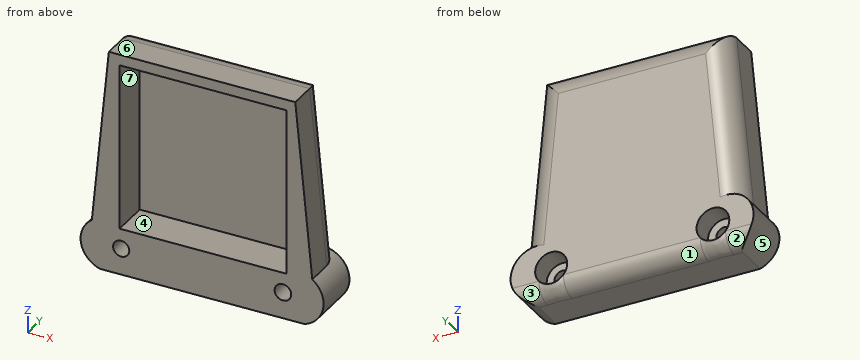
from build123d import *

# Parameters (mm, degrees)
SKETCH_R        = 1.501869
SKETCH_R_2      = 1.541907
PAD_DEPTH       = 9
SKETCH003_W     = 31
SKETCH003_H     = 31
POCKET_DEPTH    = 7
FILLET_R        = 4
SKETCH004_R     = 2.968472
SKETCH004_R_2   = 3.036595
POCKET001_DEPTH = 4
FILLET001_R     = 3


with BuildPart() as part:
    # Sketch → Pad (new body)
    with BuildSketch(Plane.XZ):
        with BuildLine():
            ThreePointArc((2.716597, 148.883863), (0.695773, 143.988618), (4.206694, 140.023699))
            Line((4.206694, 140.023699), (42.11266, 140.023699))
            ThreePointArc((42.11266, 140.023699), (45.623581, 143.988618), (43.602757, 148.883863))
            Line((40.447369, 181.653), (43.602757, 148.883863))
            Line((5.871985, 181.653), (40.447369, 181.653))
            Line((2.716597, 148.883863), (5.871985, 181.653))
        make_face()
        with Locations((8.159677, 144.938485)):
            Circle(SKETCH_R, mode=Mode.SUBTRACT)
        with Locations((38.159677, 144.938485)):
            Circle(SKETCH_R_2, mode=Mode.SUBTRACT)
    extrude(amount=PAD_DEPTH)

    # Sketch003 (on Face10 of Pad) → Pocket (cut)
    with BuildSketch(Plane.XZ.offset(9)):
        with Locations((23.362282, 164.148895)):
            Rectangle(SKETCH003_W, SKETCH003_H)
    extrude(amount=-POCKET_DEPTH, mode=Mode.SUBTRACT)

    # Fillet
    fillet_edges = [part.edges().sort_by_distance(p)[0] for p in [
        (42.025063, 0, 165.268432),
        (23.159677, 0, 181.653),
        (4.294291, 0, 165.268432),
    ]]
    fillet(fillet_edges, radius=FILLET_R)

    # Sketch004 (on Face5 of Fillet) → Pocket001 (cut)
    with BuildSketch(Plane(origin=(0, 0, 0), x_dir=(1, 0, 0), z_dir=(0, 1, 0))):
        with Locations((38.159676, -144.938507)):
            Circle(SKETCH004_R)
        with Locations((8.159677, -144.938507)):
            Circle(SKETCH004_R_2)
    extrude(amount=-POCKET001_DEPTH, mode=Mode.SUBTRACT)

    # Fillet001
    fillet001_edges = [part.edges().sort_by_distance(p)[0] for p in [
        (23.159677, 0, 140.023699),
    ]]
    fillet(fillet001_edges, radius=FILLET001_R)


solid = part.part
Input: part model. Units: mm. Frame: model coordinates. Face numbers are marked on the shaded views. A direction names the side the tool comes from. Give positions to 0.01 mm unless a question says otherwise; leave off trailing zeros. Loops run counter-clockwise (first coordinate to the right, second up) from the corner with the lowest first, then second, coordinate; pieces in that order, holes last. Notation, with made-up numbers: (23, 27) -> (54, 27) arc R23 ccw to (54, 53) -> close; hole circle Ø5 at (-39, 3). An arc over 180 degrees is marked (long way). Answer as a JSON object with one key per item and string values. Group by question number.
Item 1: Cut plane D-D, the plane y = -1. State how many separate pieces and enclosed holes the cut face has, and give its area (3 significant figures).
Item 2: Pull-direction query (Z, two-part tool) for the marked faces 5, 6 and 7; classes: released by +Z, released by -Z, zero draft, split by the parting line, or undercut.
Item 3: Cut plane B-B, the plane x = 20. Return the cut outline in (y, z).
Item 4: Pin query (flat end, axial travel): P1, Ø5.5, axis at x = 38.16, z = 144.94, coming from the +Y side; P2, Ø5, axis at y = -7, z = 177.5, coming from the -X side; P3, Ø3, axis at x = 30, z = 175, coming from the -Y side. Return the tip coordinate at first contact, or that it passes through.
Item 5: Cut plane A-A, the plane y = -8. Return the cut outline in (x, z).
Item 6: Reachability of the marked faces 1, 2, 3 and 4 from +Z, -Z, +X, -X, +Y, -Y: full face, straight path, thin tool, end or side. Return the list, or none.
Item 7: Cut plane C-C, the plane y = -3.5. Return the cut outline in (x, z), and give its area (3 significant figures).
Item 8: Line query: probe 1 along Z at (x, y) = (38, -8.25); probe 2 along X at (y, z) = (-5.25, 144); probe 3 along X at (y, z) = (-3.5, 146.5). Output: solid intervals per line, ascending.
Checks:
{
 "1": {"separate pieces": "1", "enclosed holes": "2", "area": "1,400 mm²"},
 "2": {"face 5": "split by the parting line", "face 6": "released by +Z", "face 7": "undercut"},
 "3": {"outline": "(-9, 140.02) -> (-3, 140.02) arc R3 ccw to (0, 143.02) -> (0, 177.65) arc R4 ccw to (-4, 181.65) -> (-9, 181.65) -> (-9, 179.65) -> (-2, 179.65) -> (-2, 148.65) -> (-9, 148.65) -> close"},
 "4": {"P1": "stops at y = -4", "P2": "stops at x = 5.23", "P3": "stops at y = -2"},
 "5": {"outline": "(2.72, 148.88) arc R5 ccw to (4.21, 140.02) -> (42.11, 140.02) arc R5 ccw to (43.6, 148.88) -> (40.45, 181.65) -> (5.87, 181.65) -> close; hole circle Ø3 at (8.16, 144.94); hole (7.86, 148.65) -> (38.86, 148.65) -> (38.86, 179.65) -> (7.86, 179.65) -> close; hole circle Ø3.08 at (38.16, 144.94)"},
 "6": {"face 1": "-Z, +Y", "face 2": "-Z, -X, +Y", "face 3": "-Z, +X, +Y", "face 4": "-Y"},
 "7": {"outline": "(2.75, 148.91) arc R5 ccw to (4.21, 140.02) -> (42.11, 140.02) arc R5 ccw to (43.57, 148.91) -> (40.42, 181.62) -> (5.9, 181.62) -> close; hole circle Ø6.07 at (8.16, 144.94); hole (7.86, 148.65) -> (38.86, 148.65) -> (38.86, 179.65) -> (7.86, 179.65) -> close; hole circle Ø5.94 at (38.16, 144.94)", "area": "601 mm²"},
 "8": {"probe 1": "z = 140.02 to 143.4, 146.47 to 148.65, 179.65 to 181.65", "probe 2": "x = 0.69 to 6.99, 9.33 to 36.94, 39.38 to 45.63", "probe 3": "x = 0.92 to 5.56, 10.76 to 35.64, 40.68 to 45.4"}
}
